Work out the finished part from the listing and answer in its coordinate system (mm). A direction names the side the tool comes from. Round coordinates to 2 decimals unless told otherwise and drop trailing zeros. Loops run counter-clockwise (first coordinate to the right, second up) from the corner with the lowest first, then second, coordinate; pieces in that order, holes last. Notation, with made-up numbers: (14.5, 47.5) - (23.5, 47.5) arc R35 ccw to (23.5, 83.5) - close; hole circle Ø8 at (9.5, 1). An arc over 180 degrees is marked (long way). Return JSON: item names as keys, results as strings.
Autodesk Inventor part; units mm, degrees
ref_plane "YZ Plane" through (0, 0, 0) normal (1, 0, 0) x (0, 1, 0)
ref_plane "XZ Plane" through (0, 0, 0) normal (0, 1, 0) x (-1, 0, 0)
ref_plane "XY Plane" through (0, 0, 0) normal (0, 0, 1) x (1, 0, 0)
sketch "Sketch1" plane through (0, 0, 0) normal (0, 1, 0) x (-1, 0, 0)
  line L0 (16.4526, 29.5814) -> (-36.8874, 29.5814)
  line L1 (-36.8874, 29.5814) -> (-36.8874, -38.9986)
  line L2 (-36.8874, -38.9986) -> (16.4526, -38.9986)
  line L3 (16.4526, -38.9986) -> (16.4526, 29.5814)
  point P0 (0, 0)
  dimension "d0" = 68.58
  dimension "d1" = 53.34
extrude "Extrusion1" add sketch "Sketch1" along normal blind 2.54
sketch "Sketch2" plane through (0, 0, 0) normal (0, -1, 0) x (1, 0, 0)
  line L0 (-26.6126, -49.1586) -> (47.0474, -49.1586)
  line L1 (47.0474, -49.1586) -> (47.0474, 39.7414)
  line L2 (47.0474, 39.7414) -> (-26.6126, 39.7414)
  line L3 (-26.6126, 39.7414) -> (-26.6126, -49.1586)
  line L4 (-16.4526, -38.9986) -> (-16.4526, 29.5814)
  line L5 (36.8874, 29.5814) -> (36.8874, -38.9986)
  line L6 (-16.4526, 29.5814) -> (36.8874, 29.5814)
  line L7 (36.8874, -38.9986) -> (-16.4526, -38.9986)
  point P0 (0, 0)
  dimension "d4" = 10.16
  dimension "d5" = 10.16
  dimension "d6" = 10.16
  dimension "d7" = 10.16
extrude "Extrusion2" add sketch "Sketch2" against normal blind 5.08
sketch "Sketch3" plane through (0, 5.08, 0) normal (0, 1, 0) x (1, 0, 0)
  line L0 (-26.6126, -39.7414) -> (47.0474, -39.7414)
  line L1 (-26.6126, 49.1586) -> (-26.6126, -39.7414)
  line L2 (47.0474, 49.1586) -> (-26.6126, 49.1586)
  line L3 (47.0474, -39.7414) -> (47.0474, 49.1586)
  point P0 (0, 0)
  point P1 (-21.5326, -34.6614)
  point P2 (41.9674, -34.6614)
  point P3 (41.9674, 44.0786)
  point P4 (-21.5326, 44.0786)
  dimension "d10" = 5.08
  dimension "d11" = 5.08
  dimension "d12" = 0
  dimension "d13" = 5.08
  dimension "d14" = 0
  dimension "d15" = 0
  dimension "d16" = 5.08
  dimension "d17" = 0
hole "Hole1" at (-21.5326, 5.08, 34.6614) at (41.9674, 5.08, 34.6614) at (41.9674, 5.08, -44.0786) at (-21.5326, 5.08, -44.0786) direction (0, -1, 0) diameter 5.08 depth 25.4 tip angle 118
sketch "Sketch4" plane through (0, 2.54, 0) normal (0, 1, 0) x (1, 0, 0)
  circle A0 centre (-14.2126, -15.5814) radius 5.08
  circle A1 centre (33.5874, -16.6814) radius 5.08
  circle A2 centre (28.8874, 35.2186) radius 5.08
  circle A3 centre (0.9874, 35.2186) radius 5.08
  line L0 (36.8874, 38.9986) -> (36.8874, -29.5814)
  line L1 (-26.6126, -39.7414) -> (47.0474, -39.7414)
  line L2 (36.8874, -29.5814) -> (-16.4526, -29.5814)
  line L3 (-16.4526, -29.5814) -> (-16.4526, 38.9986)
  point P0 (0, 0)
  dimension "d25" = 10.16
  dimension "d26" = 10.16
  dimension "d27" = 10.16
  dimension "d28" = 10.16
  dimension "d36" = 27.9
  dimension "d41" = 51.9
  dimension "d42" = 50.8
  dimension "d43" = 15.2
  dimension "d44" = 0
  dimension "d45" = 3.3
  dimension "d46" = 4.7
  dimension "d47" = 14
extrude "Extrusion3" add sketch "Sketch4" along normal blind 5.08
sketch "Sketch5" plane through (0.9874, 7.62, -35.2186) normal (0, 1, 0) x (1, 0, 0)
  point P0 (-0.9874, -35.2186)
  point P1 (0, 0)
hole "Hole2" at (0.9874, 7.62, -35.2186) direction (0, -1, 0) diameter 1.778 depth 25.4 tip angle 118
sketch "Sketch6" plane through (28.8874, 7.62, -35.2186) normal (0, 1, 0) x (1, 0, 0)
  point P0 (-28.8874, -35.2186)
  point P1 (0, 0)
hole "Hole3" at (28.8874, 7.62, -35.2186) direction (0, -1, 0) diameter 1.778 depth 25.4 tip angle 118
sketch "Sketch7" plane through (33.5874, 7.62, 16.6814) normal (0, 1, 0) x (1, 0, 0)
  point P0 (-33.5874, 16.6814)
  point P1 (0, 0)
hole "Hole4" at (33.5874, 7.62, 16.6814) direction (0, -1, 0) diameter 1.778 depth 25.4 tip angle 118
sketch "Sketch8" plane through (-14.2126, 7.62, 15.5814) normal (0, 1, 0) x (1, 0, 0)
  point P0 (14.2126, 15.5814)
  point P1 (0, 0)
hole "Hole5" at (-14.2126, 7.62, 15.5814) direction (0, -1, 0) diameter 1.778 depth 25.4 tip angle 118
properties part number "ArduinoMount"
1) Flat-ended cylindrical pins translate along their axes: pin 1 (2 mm diameter, centred on x = 0.99, z = -35.22, fed in from +Y); pin 2 (16 mm diameter, centred on x = 1.5, z = 3.5, fed in from +Y); pin 3 (12 mm diameter, centred on x = 31.5, z = -11, fed in from +Y). Find the tip coordinate at first contact, or state that the pin passes through.
Verdict:
{"pin 1": "stops at y = 7.62", "pin 2": "stops at y = 2.54", "pin 3": "stops at y = 5.08"}
2) Section D-D (x = -20.5) is taken. Give the vertices of the cut face in (y, z).
Verdict:
{"outline": "(0, -49.16) - (5.08, -49.16) - (5.08, -46.4) - (0, -46.4) - close; (0, -41.76) - (5.08, -41.76) - (5.08, 32.34) - (0, 32.34) - close; (0, 36.98) - (5.08, 36.98) - (5.08, 39.74) - (0, 39.74) - close"}
3) Section B-B (z = 28.5) is taken. Give the vertices of the cut face in (x, y), and give its area (3 significant figures).
Verdict:
{"outline": "(-26.61, 0) - (47.05, 0) - (47.05, 5.08) - (36.89, 5.08) - (36.89, 2.54) - (-16.45, 2.54) - (-16.45, 5.08) - (-26.61, 5.08) - close", "area": "239 mm2"}
4) Find the intervals of material crossed by L1, parallel to Z at x = -8.5, y = 3.5; L2, parallel to Z at x = -14, y = 4.25; L3, parallel to X at y = 2.75, z = -13, in increasing order.
Verdict:
{"L1": "z = -49.16 to -39, 29.58 to 39.74", "L2": "z = -49.16 to -39, 10.51 to 14.72, 16.44 to 20.66, 29.58 to 39.74", "L3": "x = -26.61 to -16.45, 36.89 to 47.05"}
5) A tool of negligible diameter and unlimited length cuts with its end or side. For faces 3 (the flat face through (10, 4, 29.581)), 4 (the flat face through (30, 7.62, -35)), from which of +Z, -Z, +X, -X, +Y, -Y can it reach the whole face along a straight path? Write none if from no direction.
Verdict:
{"face 3": "+Y", "face 4": "+Z, -Z, +X, -X, +Y"}
6) Section A-A (x = -6.5) is taken. Give the vertices of the cut face in (y, z).
Verdict:
{"outline": "(0, -49.16) - (5.08, -49.16) - (5.08, -39) - (2.54, -39) - (2.54, 29.58) - (5.08, 29.58) - (5.08, 39.74) - (0, 39.74) - close"}
7) Determine the mould class of faces 1 (the flat face through (34, 7.62, 18)), 2 (the cylindrical face through (-9.37, 5.04, 17.11)) for opening direction X: pulls with the +X half, pulls with the -X half, needs draft (parallel to the pull), parting line crosses it, or undercut.
Verdict:
{"face 1": "needs draft", "face 2": "undercut"}
8) Section C-C (y = 4) is taken. Count the separate pieces of the cut face and the enclosed holes in it, and give its area (3 significant figures).
Verdict:
{"separate pieces": "1", "enclosed holes": "9", "area": "3,080 mm2"}
